Can you work these out from the model? Positions are in its coordinate system, mm. Give positions to 0.01 mm unless a question says otherwise; leave off trailing zeros. Order: outer loops, then holes, each group sorted by start corner. A loop starts at its lowest first (then second) coordinate and runs counter-clockwise, first axis right, second up.
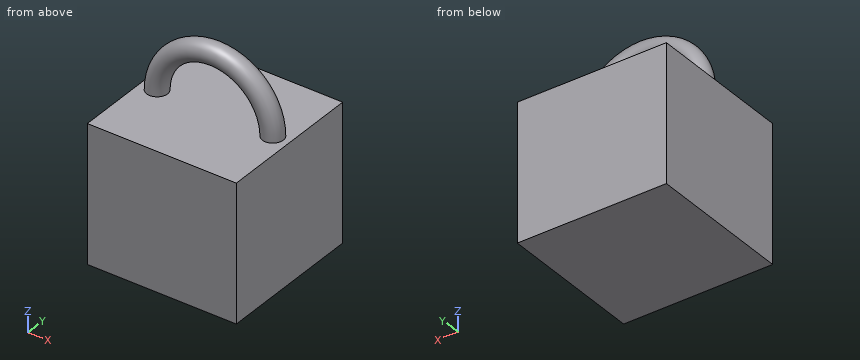
```python
from build123d import *

# Parameters (mm, degrees)
F1_R     = 9.824635
F0_W     = 69.863096
F0_H     = 137.526572
F3_DEPTH = 128.27


with BuildPart() as f2:
    # F1 (on Top) → F2 (revolve)
    with BuildSketch(Plane.XY):
        with Locations((54.264009, 0)):
            Circle(F1_R)
    revolve(axis=Axis((0, 0, 0), (0, -1, 0)))

    # F0 (on Top) → F3 (join)
    with BuildSketch(Plane.XY):
        with Locations((-34.931548, 0)):
            Rectangle(F0_W, F0_H)
        with Locations((34.931548, 0)):
            Rectangle(F0_W, F0_H)
    extrude(amount=-F3_DEPTH)


solid = f2.part
```
1) If I drill on line 1 (Z direction, x = 64, y = -15); line 2 (X direction, y = 6, z = 22); line 3 (X direction, y = 8, z = 26.5), over which ranges is the centre line in solid material (lowest first)?
2) I'm going to push flat-ended pins straight in: pin 1 Ø4 at (x, y) = (-51, -37.5) entering from +Z; pin 2 Ø12 at (x, y) = (42, -12) entering from +Z. Where does each tip first touch, or does it pass through?
3) Suppose I cut it at A-A (y = 34). Please give me the cut outline in (x, z), and give its area (3 significant figures).
Results:
1. line 1: z = -128.27 to 0
1. line 2: x = -58.01 to -40.95, 40.95 to 58.01
1. line 3: x = -53.79 to -40.69, 40.69 to 53.79
2. pin 1: stops at z = 0
2. pin 2: stops at z = 47.37
3. outline: (-69.86, -128.27) - (69.86, -128.27) - (69.86, 0) - (-69.86, 0) - close
3. area: 17,900 mm2
